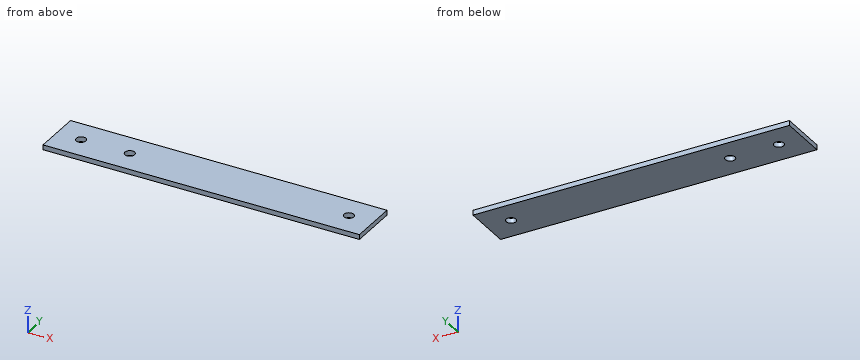
```python
from build123d import *

# Parameters (mm, degrees)
SKETCH1_W           = 130
SKETCH1_H           = 20
BOSS_EXTRUDE1_DEPTH = 2
SKETCH2_R           = 2
CUT_EXTRUDE1_DEPTH  = 2
SKETCH3_R           = 2
CUT_EXTRUDE2_DEPTH  = 2


with BuildPart() as part:
    # Sketch1 → Boss-Extrude1 (new body)
    with BuildSketch(Plane.XY):
        Rectangle(SKETCH1_W, SKETCH1_H)
    extrude(amount=BOSS_EXTRUDE1_DEPTH)

    # Sketch2 → Cut-Extrude1 (cut)
    with BuildSketch(Plane.XY.offset(2)):
        with Locations((-55, 0)):
            Circle(SKETCH2_R)
        with Locations((55, 0)):
            Circle(SKETCH2_R)
    extrude(amount=-CUT_EXTRUDE1_DEPTH, mode=Mode.SUBTRACT)

    # Sketch3 → Cut-Extrude2 (cut)
    with BuildSketch(Plane.XY.offset(2)):
        with Locations((-35, 0)):
            Circle(SKETCH3_R)
    extrude(amount=-CUT_EXTRUDE2_DEPTH, mode=Mode.SUBTRACT)


solid = part.part
```
Verification items for the finished model (mm, model axes). Coordinates: 2 decimals unless noted, no trailing zeros. Order: outer loops, then holes, each group sorted by start corner. A loop starts at its lowest first (then second) coordinate and runs counter-clockwise, first axis right, second up. Notation, with made-up numbers: (16, 32.25) -> (72, 32.25) arc R8 cw to (72, 46.25) -> close; hole circle Ø5 at (50.25, -19.75). An arc over 180 degrees is marked (long way). Answer as CSV lines item,"result". Start each with the question number.
1) Cross-section at A-A, the plane x = -55. Record the boundary of the cut face in (y, z).
2) Material ranges on L1, parallel to X at y = 0.25, z = 0.75; L2, parallel to Y at x = -35, z = 1.55, recorded low to high. Write a range as [from, to].
3) Gauge pin test, flat ends, axial feed: pin 1 Ø6.5 at (x, y) = (-35, 0) entering from -Z; pin 2 Ø2.5 at (x, y) = (-55, 0) entering from -Z. Record the tip position at first contact, or that the pin passes through.
Conclusion:
1,outline,"(-10, 0) -> (-2, 0) -> (-2, 2) -> (-10, 2) -> close; (2, 0) -> (10, 0) -> (10, 2) -> (2, 2) -> close"
2,L1,"x = [-65, -56.98], [-53.02, -36.98], [-33.02, 53.02], [56.98, 65]"
2,L2,"y = [-10, -2], [2, 10]"
3,pin 1,"stops at z = 0"
3,pin 2,"passes through"
